```python
from build123d import *

# Parameters (mm, degrees)
BOSS_EXTRUDE1_DEPTH = 80
SKETCH2_W           = 30
SKETCH2_H           = 5
BOSS_EXTRUDE2_DEPTH = 13
SKETCH3_W           = 30
SKETCH3_H           = 12.5
BOSS_EXTRUDE3_DEPTH = 5


with BuildPart() as part:
    # Sketch1 → Boss-Extrude1 (new body)
    with BuildSketch(Plane(origin=(0, 0, 0), x_dir=(0, 0, -1), z_dir=(1, 0, 0))):
        Polygon((0, 10), (42.261826174, 100.630778704), (46.074889763, 92.453637449), (71.431985467, 38.075170227), (63.645988922, 38.075170227), (43.368827902, 81.559682364), (10, 10), (90, 10), (90, 0), (0, 0), align=None)
    extrude(amount=BOSS_EXTRUDE1_DEPTH)

    # Sketch2 → Boss-Extrude2 (add)
    with BuildSketch(Plane(origin=(0, 34.160499048, -73.257426617), x_dir=(-1, 0, 0), z_dir=(0, 0.4226182617406983, -0.9063077870366506))):
        with Locations((-65, 6.819361739)):
            Rectangle(SKETCH2_W, SKETCH2_H)
        with Locations((-15, 6.819361739)):
            Rectangle(SKETCH2_W, SKETCH2_H)
    extrude(amount=BOSS_EXTRUDE2_DEPTH)

    # Sketch3 → Boss-Extrude3 (add)
    with BuildSketch(Plane(origin=(0, 39.654536451, -85.039427849), x_dir=(-1, 0, 0), z_dir=(0, 0.4226182617406977, -0.9063077870366508))):
        with Locations((-65, 10.569361739)):
            Rectangle(SKETCH3_W, SKETCH3_H)
        with Locations((-15, 10.569361739)):
            Rectangle(SKETCH3_W, SKETCH3_H)
    extrude(amount=BOSS_EXTRUDE3_DEPTH)


solid = part.part
```
Could you check a few things on this model? Use its own coordinates, in mm. A direction names the side the tool comes from. Coordinates: 2 decimals unless noted, no trailing zeros. Write each loop counter-clockwise with the first axis right and the second up, starting at its lowest first coordinate (ties: lowest second). Pieces come first, ordered by that corner, then holes. Notation, with made-up numbers: (4.25, 0) -> (38.25, 0) arc R22 ccw to (38.25, 15) -> close; hole circle Ø3 at (-28.75, 68.25). An arc over 180 degrees is marked (long way). Return JSON: item names as keys, results as strings.
(1) Imagine slicing it at D-D, the plane y = 71.5. Please give me the cut outline in (x, z), then the cut area to 3 significant figures.
Numbers:
{"outline": "(0, -55.85) -> (80, -55.85) -> (80, -48.06) -> (0, -48.06) -> close; (0, -38.68) -> (80, -38.68) -> (80, -28.68) -> (0, -28.68) -> close", "area": "1,420 mm2"}
(2) Which directions (+Z, -Z, +X, -X, +Y, -Y) give clear straight access to the entire face, cutting with the end or side of a thin tool? Please do faces 1 (the flat face through (39, 5, 0)), 2 (the flat face through (65.21, 55.94, -80.17)), 3 (the flat face through (65.21, 45.315, -75.127)), 4 (the flat face through (65.21, 41.825, -79.475)), 5 (the flat face through (65.21, 51.426, -85.067)).
Numbers:
{"face 1": "+Z, +X, -X, +Y, -Y", "face 2": "+X, -X, +Y", "face 3": "+X, -X", "face 4": "-Z, +X, -X", "face 5": "-Z, +X, -X, +Y"}
(3) Imagine slicing it at A-A, the plane z = -17. Please give me the cut outline in (x, y), then the cut area to 3 significant figures.
Numbers:
{"outline": "(0, 0) -> (80, 0) -> (80, 10) -> (0, 10) -> close; (0, 25.01) -> (80, 25.01) -> (80, 46.46) -> (0, 46.46) -> close", "area": "2,520 mm2"}
(4) Imagine slicing it at C-C, the plane z = -74. Please give me the cut outline in (x, y).
Numbers:
{"outline": "(0, 0) -> (80, 0) -> (80, 10) -> (0, 10) -> close; (0, 39.27) -> (30, 39.27) -> (30, 44.79) -> (0, 44.79) -> close; (50, 39.27) -> (80, 39.27) -> (80, 44.79) -> (50, 44.79) -> close"}
(5) Imagine slicing it at B-B, the plane x = 5. Please give me the cut outline in (y, z).
Numbers:
{"outline": "(0, -90) -> (10, -90) -> (10, -10) -> (81.56, -43.37) -> (38.08, -63.65) -> (38.08, -71.43) -> (45.68, -87.75) -> (57.01, -82.46) -> (54.9, -77.93) -> (48.1, -81.1) -> (42.61, -69.32) -> (100.63, -42.26) -> (10, 0) -> (0, 0) -> close"}
(6) I need wall thicknesses on L1, parallel to Z at x = 76, y = 53.5; L2, parallel to Z at x = 45.5, y = 45; L3, parallel to Y at x = 41, z = -48. Which ranges of each line are inside material? Lowest first, please.
Numbers:
{"L1": "z = -84.1 to -78.58, -64.24 to -56.45, -30.28 to -20.28", "L2": "z = -68.2 to -60.42, -26.32 to -16.32", "L3": "y = 0 to 10, 71.63 to 88.33"}
(7) We'd pull the mould along Y, two halves only. Please class faces 6 (the flat face through (39, 0, -46)), 7 (the flat face through (15.21, 51.426, -85.067)), 8 (the flat face through (65.21, 51.547, -79.494)), 9 (the flat face through (0, 43, -25)): +Y half, -Y half, draft (parallel to the pull), parting line (faces both ways), or undercut.
Numbers:
{"face 6": "-Y half", "face 7": "+Y half", "face 8": "undercut", "face 9": "draft"}
(8) I'm going to push flat-ended pins straight in: pin 1 (8 mm diameter, centred on x = 63.5, z = -11.5, fed in from +Y); pin 2 (1.5 mm diameter, centred on x = 14.5, y = 18.5, fed in from +Z); pin 3 (4 mm diameter, centred on x = 30.5, y = 50, fed in from -Z). Where does each tip first touch, or does it pass through?
Numbers:
{"pin 1": "stops at y = 43.24", "pin 2": "stops at z = -3.61", "pin 3": "stops at z = -86.64"}
